The listing builds one solid part. Answer for the finished solid, in the listing's coordinates (mm). Face numbers are marked on the shaded views. A direction names the side the tool comes from. Coordinates: 2 decimals unless noted, no trailing zeros. Order: outer loops, then holes, each group sorted by start corner. A loop starts at its lowest first (then second) coordinate and runs counter-clockwise, first axis right, second up. Notation, with made-up numbers: (-23.75, 81) -> (-17.75, 81) arc R13 cw to (-17.75, 95) -> close; hole circle Ø10 at (87.5, 45.5). An arc over 180 degrees is marked (long way). Write item = value, one per line.
from build123d import *

# Parameters (mm, degrees)
SKETCH_1_R      = 15
EXTRUDE_1_DEPTH = 30
EXTRUDE_2_DEPTH = 12
SKETCH_9_R      = 3
EXTRUDE_3_DEPTH = 14.5


with BuildPart() as part:
    # 草图1 → 凸台-拉伸1 (new body)
    with BuildSketch(Plane(origin=(0, 0, 0), x_dir=(0, 0, -1), z_dir=(1, 0, 0))):
        Circle(SKETCH_1_R)
    extrude(amount=-EXTRUDE_1_DEPTH)

    # 草图8 → 凸台-拉伸2 (add)
    with BuildSketch(Plane(origin=(0, 0, 0), x_dir=(0, 0, -1), z_dir=(1, 0, 0))):
        with BuildLine():
            Line((19, 10.6), (19, -33.9))
            ThreePointArc((19, -33.9), (16.071067812, -40.971067812), (9, -43.9))
            Line((9, -43.9), (-9, -43.9))
            ThreePointArc((-9, -43.9), (-16.071067812, -40.971067812), (-19, -33.9))
            Line((-19, -33.9), (-19, 10.6))
            ThreePointArc((-19, 10.6), (-16.071067812, 17.671067812), (-9, 20.6))
            Line((-9, 20.6), (9, 20.6))
            ThreePointArc((9, 20.6), (16.071067812, 17.671067812), (19, 10.6))
        make_face()
    extrude(amount=EXTRUDE_2_DEPTH)

    # 草图9 → 凸台-拉伸3 (add)
    with BuildSketch(Plane(origin=(12, 0, 0), x_dir=(0, 0, -1), z_dir=(1, 0, 0))):
        with Locations(Location((0, -31, 0), (0, 0, 180))):
            Circle(SKETCH_9_R)
    extrude(amount=EXTRUDE_3_DEPTH)


solid = part.part
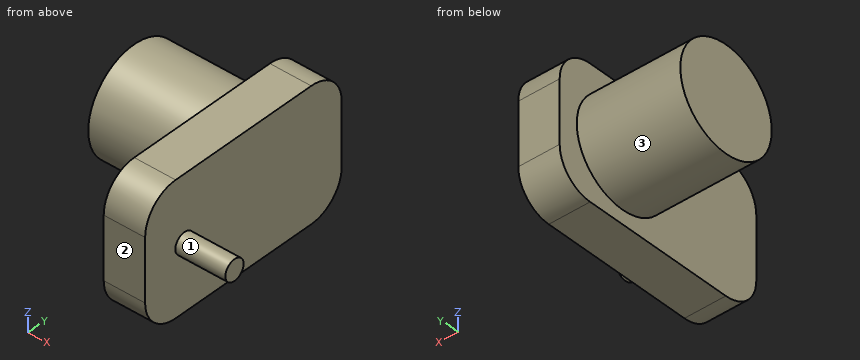
Q1. A tool of negligible diameter and unlimited length cuts with its end or side. For the marked faces 1, 2 and 3, from which of +Z, -Z, +X, -X, +Y, -Y can it reach the whole face along a straight path? Write none if from no direction.
The answers:
face_1 = +X
face_2 = +Z, -Z, +X, -X, -Y
face_3 = -X
Q2. Section D-D, the plane x = -1.5 is taken. Give the vertices of the cut face in (y, z).
The answers:
outline = circle Ø30 at (0, 0)
Q3. Each of these flat-tipped pins is pushed along its axis until it touches: pin 1 Ø19 at (y, z) = (-26.5, -4) entering from -X; pin 2 Ø12 at (x, y) = (15, -9) entering from +Z; pin 3 Ø5 at (x, y) = (-23.5, -7) entering from +Z; pin 4 Ø2 at (x, z) = (15, -3) entering from -Y. Where does it stop, or does it pass through?
The answers:
pin_1 = 0
pin_2 = 19
pin_3 = 14.31
pin_4 = -33.24
Q4. Section C-C, the plane z = 0 is taken. Give the vertices of the cut face in (x, y).
The answers:
outline = (-30, -15) -> (0, -15) -> (0, -43.9) -> (12, -43.9) -> (12, -34) -> (26.5, -34) -> (26.5, -28) -> (12, -28) -> (12, 20.6) -> (0, 20.6) -> (0, 15) -> (-30, 15) -> close
Q5. Section B-B, the plane x = 5.5 is taken. Give the vertices of the cut face in (y, z), plus the area to 3 significant figures.
The answers:
outline = (-43.9, -9) arc R10 ccw to (-33.9, -19) -> (10.6, -19) arc R10 ccw to (20.6, -9) -> (20.6, 9) arc R10 ccw to (10.6, 19) -> (-33.9, 19) arc R10 ccw to (-43.9, 9) -> close
area = 2,370 mm2
Q6. Section A-A, the plane y = -31 is taken. Give the vertices of the cut face in (x, z).
The answers:
outline = (0, -19) -> (12, -19) -> (12, -3) -> (26.5, -3) -> (26.5, 3) -> (12, 3) -> (12, 19) -> (0, 19) -> close
Q7. Find the intervals of material crossed by line 1 along X through (y, z) = (-11.5, 1.5); line 2 along X through (y, z) = (-32, 6.5); line 3 along Z through (x, y) = (-5.5, -4.5), in increasing order.
The answers:
line_1 = -30 to 12
line_2 = 0 to 12
line_3 = -14.31 to 14.31
